Design review of the part built by this model. Coordinates are the model's own, in mm. Give positions to 0.01 mm unless a question says otherwise; leave off trailing zeros. Loops run counter-clockwise (first coordinate to the right, second up) from the corner with the lowest first, then second, coordinate; pieces in that order, holes last. Notation, with made-up numbers: (-23, -21) -> (36, -21) arc R24 cw to (36, -8) -> close; hole circle Ø4 at (15, 30). An arc over 180 degrees is marked (long way). Answer in a Markdown table with one row per item. Add a question column.
(1) Consider section C-C on z = 1.75. Write out the cut boundary in (x, y), then the cut area to 3 significant figures.
(2) For line 1 (Y direction, x = 0, z = 4.25); line 2 (X direction, y = -1, z = 4.5); line 3 (X direction, y = -0.75, z = 9), list the stretches that pass through material, from the lowest coordinate up.
(3) Draft analysis for pull direction Y (two halves, no side actions). For faces 1 (the cylindrical face through (-2.9, 0.1, 5.3)), 2 (the flat face through (-1, 3, 0)), 3 (the cylindrical face through (3.233, -1.341, 4.881)), state which applies: +Y half, -Y half, draft (parallel to the pull), parting line (faces both ways), or undercut.
(4) For pin 1 (3.5 mm diameter, centred on x = -0.5, y = -1, fed in from -Z); pin 2 (3 mm diameter, centred on y = 3, z = 2.5, fed in from +X), all flat-tipped, find the tip position at first contact; note any pin that passes through.
from build123d import *

# Parameters (mm, degrees)
ESQUISSE1_R          = 3.5
ESQUISSE1_R_2        = 2.9
BASE_EXTRUSION_DEPTH = 11
ESQUISSE2_W          = 0.6
ESQUISSE2_H          = 0.25
CONG_3_R             = 0.3


with BuildPart() as part:
    # Esquisse1 → Base-Extrusion (new body)
    with BuildSketch(Plane.XY):
        Circle(ESQUISSE1_R)
        Circle(ESQUISSE1_R_2, mode=Mode.SUBTRACT)
    extrude(amount=BASE_EXTRUSION_DEPTH)

    # Esquisse2 → Enlèvement de matière-Révolution1 (revolve, cut)
    with BuildSketch(Plane(origin=(0, 0, 0), x_dir=(0, 0, -1), z_dir=(1, 0, 0)), mode=Mode.PRIVATE) as enl_vement_de_mati_re_r_volution1_sk:
        with Locations((-10.2, 3.375)):
            Rectangle(ESQUISSE2_W, ESQUISSE2_H)
    revolve(enl_vement_de_mati_re_r_volution1_sk.sketch.rotate(Axis((0, 0, 10), (0, 0, -1)), 90), axis=Axis((0, 0, 10), (0, 0, -1)), mode=Mode.SUBTRACT)

    # Congé3
    cong_3_edges = [part.edges().sort_by_distance(p)[0] for p in [
        (-2.9, 0, 11),
        (-3.5, 0, 11),
    ]]
    fillet(cong_3_edges, radius=CONG_3_R - 0.0001)  # a hair under: the kernel refuses the full size


solid = part.part
Values follow:
| question | item | result |
|---|---|---|
| 1 | outline | circle Ø7 at (0, 0); hole circle Ø5.8 at (0, 0) |
| 1 | area | 12.1 mm2 |
| 2 | line 1 | -3.5 to -2.9, 2.9 to 3.5 |
| 2 | line 2 | -3.35 to -2.72, 2.72 to 3.35 |
| 2 | line 3 | -3.42 to -2.8, 2.8 to 3.42 |
| 3 | face 1 | undercut |
| 3 | face 2 | draft |
| 3 | face 3 | parting line |
| 4 | pin 1 | through |
| 4 | pin 2 | x = 3.16 |
